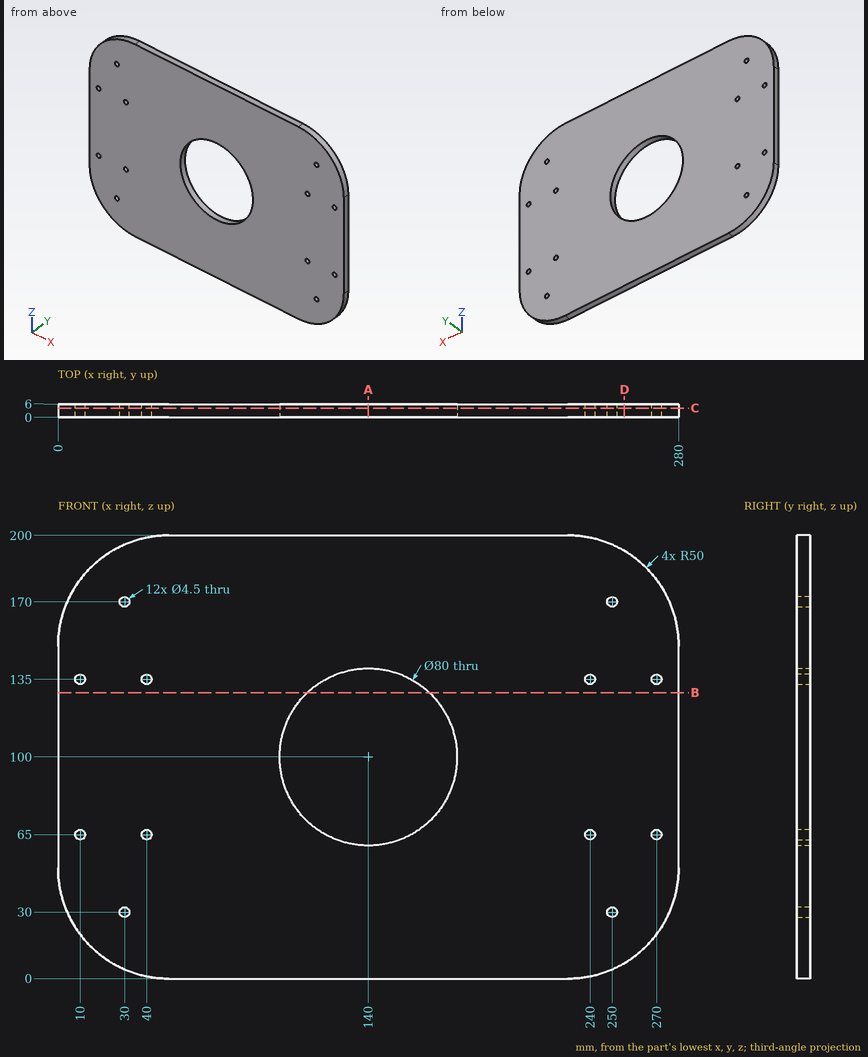
The drawing under review shows one solid part. Ordinate dimensions are in mm from its lowest x, y, z. Give positions to 0.01 mm unless a question says otherwise; leave off trailing zeros. Order: outer loops, then holes, each group sorted by start corner. A loop starts at its lowest first (then second) coordinate and runs counter-clockwise, first axis right, second up. Notation, with made-up numbers: M 22,-4.75 L 71,-4.75 A22 cw 71,9.25 Z; hole C 20.5,59 d2. An arc over 180 degrees is marked long. Answer in a Markdown table with one row per item. Add a question column.
1. Add section B-B on z = 129. State the section outline as (x, y) points, plus the area to 3 significant figures.
2. For pin 1 Ø5 at (x, z) = (270, 135) entering from +Y; pin 2 Ø2 at (y, z) = (4.5, 38) entering from -X (3 decimals), all flat-tipped, find the tip position at first contact; note any pin that passes through.
3. Add section D-D on x = 255.5. State the section outline as (y, z) points, plus the area to 3 significant figures.
4. Add section A-A on x = 140. State the section outline as (y, z) points.
5. Add section C-C on y = 4.15. Count the separate pieces of the cut face and the enclosed holes in it, plus the area to 3 significant figures.
6. To check wall thickness, follow line 1 along X through (y, z) = (3.1, 135); line 2 along X through (y, z) = (4.65, 133.5); line 3 along X through (y, z) = (2.35, 30). State the ranges of each line that lie inside material, in increasing order.
The answers:
| question | item | result |
|---|---|---|
| 1 | outline | M 0,0 L 112.45,0 L 112.45,6 L 0,6 Z; M 167.55,0 L 280,0 L 280,6 L 167.55,6 Z |
| 1 | area | 1,350 mm2 |
| 2 | pin 1 | y = 6 |
| 2 | pin 2 | x = 1.225 |
| 3 | outline | M 0,6.99 L 6,6.99 L 6,193.01 L 0,193.01 Z |
| 3 | area | 1,120 mm2 |
| 4 | outline | M 0,0 L 6,0 L 6,60 L 0,60 Z; M 0,140 L 6,140 L 6,200 L 0,200 Z |
| 5 | separate pieces | 1 |
| 5 | enclosed holes | 13 |
| 5 | area | 48,600 mm2 |
| 6 | line 1 | 0 to 7.75, 12.25 to 37.75, 42.25 to 120.64, 159.36 to 237.75, 242.25 to 267.75, 272.25 to 280 |
| 6 | line 2 | 0 to 8.32, 11.68 to 38.32, 41.68 to 118.14, 161.86 to 238.32, 241.68 to 268.32, 271.68 to 280 |
| 6 | line 3 | 4.17 to 27.75, 32.25 to 247.75, 252.25 to 275.83 |
